```python
from build123d import *

# Parameters (mm, degrees)
SKETCH2_R          = 12.7
SKETCH2_R_2        = 11.2141
EXTRUDE1_DEPTH     = 28.575
SKETCH3_R          = 12.7
SKETCH3_R_2        = 9.017
EXTRUDE2_DEPTH     = 25.4
SKETCH4_R          = 11.2141
SKETCH4_R_2        = 9.017
CUT_EXTRUDE3_DEPTH = 3.175


with BuildPart() as part:
    # Sketch2 → Extrude1 (new body)
    with BuildSketch(Plane(origin=(0, 0, 0), x_dir=(0, 0, -1), z_dir=(1, 0, 0))):
        Circle(SKETCH2_R)
        Circle(SKETCH2_R_2, mode=Mode.SUBTRACT)
    extrude(amount=EXTRUDE1_DEPTH)

    # Sketch3 → Extrude2 (add)
    with BuildSketch(Plane(origin=(28.575, 0, 0), x_dir=(0, 0, -1), z_dir=(1, 0, 0))):
        Circle(SKETCH3_R)
        Circle(SKETCH3_R_2, mode=Mode.SUBTRACT)
    extrude(amount=EXTRUDE2_DEPTH)

    # Sketch4 → Cut-Extrude3 (cut)
    with BuildSketch(Plane.ZY.offset(-28.575)):
        with Locations(Location((0, 0, 0), (0, 0, 180))):  # turned: the seam where the file's is
            Circle(SKETCH4_R)
        with Locations(Location((0, 0, 0), (0, 0, 180))):  # turned: the seam where the file's is
            Circle(SKETCH4_R_2, mode=Mode.SUBTRACT)
    extrude(amount=-CUT_EXTRUDE3_DEPTH, mode=Mode.SUBTRACT)


solid = part.part
```
Check sheet for the modelled part. Datum: model origin and axes. Units: mm. A direction names the side the tool comes from. Round coordinates to 2 decimals unless told otherwise and drop trailing zeros. Write each loop counter-clockwise with the first axis right and the second up, starting at its lowest first coordinate (ties: lowest second). Pieces come first, ordered by that corner, then holes. Notation, with made-up numbers: (64.25, 7.25) -> (96.25, 7.25) arc R8 cw to (96.25, 21.25) -> close; hole circle Ø10 at (29.5, 18.25). An arc over 180 degrees is marked (long way). One line per question, with ' | ' between items. Start each with the question number.
1. Set-up check for faces 4 (the face through (42.707, -8.803, 1.955)), 5 (the face through (15.653, 3.368, -10.696)): record each of +Z, -Z, +X, -X, +Y, -Y from which the full face is reachable in a straight line by a thin tool's end or side.
2. Sectioned sample at D-D, the plane y = 10.5. Record the cut outline in (x, z) (3 decimals), then the cut area to 3 significant figures.
3. Sectioned sample at C-C, the plane x = 47.5. Record the cut outline in (y, z), then the cut area to 3 significant figures.
4. Scan lines: line 1 along Y through (x, z) = (41.75, 0); line 2 along Y through (x, z) = (21.5, 0); line 3 along Z through (x, y) = (34, -3.75). Record each from-to range of solid material in increasing order. Write a range as from..to.
5. Depth check by flat-ended pin: pin 1 (10 mm diameter, centred on x = 22, z = 6, fed in from +Y); pin 2 (2 mm diameter, centred on x = 32.5, z = -6, fed in from +Y); pin 3 (2 mm diameter, centred on x = 14, z = 10, fed in from +Y). Enter the tip coordinate at first touch or a pass-through.
6. Release check for a two-part mould opening along Y. For faces 1 (the face through (31.75, -5, 8)), 2 (the face through (0, -9, -7)), 3 (the face through (26.61, -12.4, 2.75)) record: +Y half, -Y half, draft (parallel to the pull), parting line (faces both ways), or undercut.
7. Sectioned sample at A-A, the plane y = 0. Record the cut outline in (x, z) (3 decimals), then the cut area to 3 significant figures.
Taken from the geometry:
1) face 4: +X, -X | face 5: -X
2) outline: (0, -7.144) -> (53.975, -7.144) -> (53.975, 7.144) -> (0, 7.144) -> (0, 3.938) -> (31.75, 3.938) -> (31.75, -3.938) -> (0, -3.938) -> close | area: 521 mm^2
3) outline: circle Ø25.4 at (0, 0); hole circle Ø18.03 at (0, 0) | area: 251 mm^2
4) line 1: y = -12.7..-9.02, 9.02..12.7 | line 2: y = -12.7..-11.21, 11.21..12.7 | line 3: z = -12.13..-8.2, 8.2..12.13
5) pin 1: stops at y = 12.66 | pin 2: stops at y = 11.67 | pin 3: stops at y = 8.96
6) face 1: undercut | face 2: draft | face 3: parting line
7) outline: (0, -12.7) -> (53.975, -12.7) -> (53.975, -9.017) -> (31.75, -9.017) -> (31.75, -11.214) -> (0, -11.214) -> close; (0, 11.214) -> (31.75, 11.214) -> (31.75, 9.017) -> (53.975, 9.017) -> (53.975, 12.7) -> (0, 12.7) -> close | area: 258 mm^2
